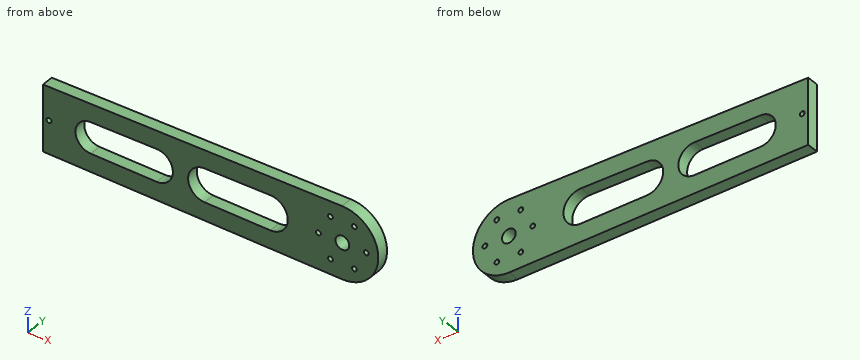
```python
from build123d import *

# Parameters (mm, degrees)
SKETCH1_R           = 5.75
SKETCH1_R_2         = 2
BOSS_EXTRUDE1_DEPTH = 10


with BuildPart() as part:
    # Sketch1 → Boss-Extrude1 (new body)
    with BuildSketch(Plane(origin=(0, 0, 0), x_dir=(1, 0, 0), z_dir=(0, 1, 0))):
        with BuildLine():
            Line((-216.382104852, 37.479356926), (33.317969978, 39.953751753))
            ThreePointArc((33.317969978, 39.953751753), (63.615239274, 9.952328714), (33.312178481, -20.043244588))
            Line((33.312178481, -20.043244588), (-216.38741399, -17.520642817))
            Line((-216.38741399, -17.520642817), (-216.382104852, 37.479356926))
        make_face()
        with Locations((33.615239414, 9.955224607)):
            Circle(SKETCH1_R, mode=Mode.SUBTRACT)
        with Locations((53.615239414, 9.955224607)):
            Circle(SKETCH1_R_2, mode=Mode.SUBTRACT)
        with Locations((43.615239414, -7.365283468)):
            Circle(SKETCH1_R_2, mode=Mode.SUBTRACT)
        with Locations((23.615239414, -7.365283468)):
            Circle(SKETCH1_R_2, mode=Mode.SUBTRACT)
        with Locations((13.615239414, 9.955224607)):
            Circle(SKETCH1_R_2, mode=Mode.SUBTRACT)
        with Locations((23.615239414, 27.275732683)):
            Circle(SKETCH1_R_2, mode=Mode.SUBTRACT)
        with Locations((43.615239414, 27.275732683)):
            Circle(SKETCH1_R_2, mode=Mode.SUBTRACT)
        with Locations((-211.384759398, 9.979356926)):
            Circle(SKETCH1_R_2, mode=Mode.SUBTRACT)
        with BuildLine():
            Line((-176.512574007, 22.873706291), (-121.518027204, 23.418672976))
            ThreePointArc((-121.518027204, 23.418672976), (-107.935613387, 9.968888481), (-121.52062356, -3.478273548))
            Line((-121.52062356, -3.478273548), (-176.515064128, -2.922689649))
            ThreePointArc((-176.515064128, -2.922689649), (-189.283603246, 9.976740986), (-176.512574007, 22.873706291))
        make_face(mode=Mode.SUBTRACT)
        with BuildLine():
            Line((-81.524666784, -3.882334565), (-26.530226217, -4.437918464))
            ThreePointArc((-26.530226217, -4.437918464), (-11.985090745, 9.959626398), (-26.527446362, 24.359979069))
            Line((-26.527446362, 24.359979069), (-81.521993165, 23.815012384))
            ThreePointArc((-81.521993165, 23.815012384), (-95.234126773, 9.967662409), (-81.524666784, -3.882334565))
        make_face(mode=Mode.SUBTRACT)
    extrude(amount=BOSS_EXTRUDE1_DEPTH)


solid = part.part
```
The listing builds one solid part. Answer for the finished solid, in the listing's coordinates (mm). Coordinates: 2 decimals unless noted, no trailing zeros. Write each loop counter-clockwise with the first axis right and the second up, starting at its lowest first coordinate (ties: lowest second). Pieces come first, ordered by that corner, then holes. Notation, with made-up numbers: (-10, 42.25) - (10, 42.25) arc R35 cw to (10, 76.25) - close; hole circle Ø7 at (-5.5, 65). An arc over 180 degrees is marked (long way). One line per item, written item: value.
1) Find section A-A (x = -185). Give the vertices of the cut face in (y, z), and give its area (3 significant figures).
Geometry check:
outline: (0, -37.79) - (10, -37.79) - (10, -19.58) - (0, -19.58) - close; (0, -0.38) - (10, -0.38) - (10, 17.84) - (0, 17.84) - close
area: 364 mm2
2) Find section C-C (z = -19). Give the vertices of the cut face in (x, y), and give its area (3 significant figures).
Geometry check:
outline: (-216.38, 0) - (-185.6, 0) - (-185.6, 10) - (-216.38, 10) - close; (-111.42, 0) - (-91.88, 0) - (-91.88, 10) - (-111.42, 10) - close; (-15.18, 0) - (62.22, 0) - (62.22, 10) - (-15.18, 10) - close
area: 1,280 mm2
3) Each of these flat-tipped pins is pushed along its axis until it touches: pin 1 Ø5 at (x, y) = (-106, 4) entering from +Z; pin 2 Ø4 at (y, z) = (8, 9.5) entering from +X; pin 3 Ø1.5 at (y, z) = (6, 5) entering from +X; pin 4 Ø2.5 at (x, z) = (23.62, 7.37) entering from +Y (3 decimals). Where does it stop, or does it pass through?
Geometry check:
pin 1: stops at z = 18.66
pin 2: stops at x = 58.01
pin 3: stops at x = 60.04
pin 4: passes through
4) Consider line 1 along X through (y, z) = (2.25, -20.5); line 2 along X through (y, z) = (6, -21.5); line 3 along X through (y, z) = (9.5, -6.5). Determine where each line is inside the solid, lowest interval first. Write a range as from..to.
Geometry check:
line 1: x = -216.38..-183.84, -113.02..-90.38, -16.57..61.7
line 2: x = -216.38..-182.18, -114.46..-89.05, -17.77..61.3
line 3: x = -216.39..-188.81, -108.39..-94.79, -12.41..29.02, 38.21..63.42
5) Find section D-D (x = -70). Give the vertices of the cut face in (y, z).
Geometry check:
outline: (0, -38.93) - (10, -38.93) - (10, -23.93) - (0, -23.93) - close; (0, 4) - (10, 4) - (10, 19) - (0, 19) - close
6) Find section B-B (y = 4.25). Count the separate pieces of the cut face and the enclosed holes in it, and give its area (3 significant figures).
Geometry check:
separate pieces: 1
enclosed holes: 10
area: 11,400 mm2
